For this review, take the finished solid that the model builds, in its own axes (mm). Give positions to 0.01 mm unless a question says otherwise; leave off trailing zeros. Write each loop counter-clockwise with the first axis right and the second up, starting at its lowest first coordinate (ties: lowest second). Pieces come first, ordered by that corner, then holes. Notation, with made-up numbers: (7.5, -33) -> (20.5, -33) arc R17 ccw to (20.5, -11) -> close; hole circle Ø10 at (88, 36). An arc over 180 degrees is marked (long way). Write item = value, one per line.
```python
from build123d import *

# Parameters (mm, degrees)
F0_R     = 1.5875
F1_DEPTH = 9
F3_W     = 12
F3_H     = 74
F4_DEPTH = 4


with BuildPart() as f1:
    # F0 (on Top) → F1 (new body)
    with BuildSketch(Plane.XY):
        Polygon((177, -37), (177, 37), (130, 37), (120, 47), (-120, 47), (-130, 37), (-177, 37), (-177, -37), (-130, -37), (-120, -47), (120, -47), (130, -37), align=None)
        with Locations((-135, -30)):
            Circle(F0_R, mode=Mode.SUBTRACT)
        with BuildLine():
            Line((-168, -8.5875), (-172, -8.5875))
            ThreePointArc((-172, -8.5875), (-173.5875, -7), (-172, -5.4125))
            Line((-172, -5.4125), (-168, -5.4125))
            ThreePointArc((-168, -5.4125), (-166.4125, -7), (-168, -8.5875))
        make_face(mode=Mode.SUBTRACT)
        with Locations((135, -30)):
            Circle(F0_R, mode=Mode.SUBTRACT)
        with BuildLine():
            Line((147, -21.4125), (151, -21.4125))
            ThreePointArc((151, -21.4125), (152.5875, -23), (151, -24.5875))
            Line((151, -24.5875), (147, -24.5875))
            ThreePointArc((147, -24.5875), (145.4125, -23), (147, -21.4125))
        make_face(mode=Mode.SUBTRACT)
        with BuildLine():
            Line((168, -13.4125), (172, -13.4125))
            ThreePointArc((172, -13.4125), (173.5875, -15), (172, -16.5875))
            Line((172, -16.5875), (168, -16.5875))
            ThreePointArc((168, -16.5875), (166.4125, -15), (168, -13.4125))
        make_face(mode=Mode.SUBTRACT)
        with BuildLine():
            Line((-168, 13.4125), (-172, 13.4125))
            ThreePointArc((-172, 13.4125), (-173.5875, 15), (-172, 16.5875))
            Line((-172, 16.5875), (-168, 16.5875))
            ThreePointArc((-168, 16.5875), (-166.4125, 15), (-168, 13.4125))
        make_face(mode=Mode.SUBTRACT)
        with BuildLine():
            Line((-147, 21.4125), (-151, 21.4125))
            ThreePointArc((-151, 21.4125), (-152.5875, 23), (-151, 24.5875))
            Line((-151, 24.5875), (-147, 24.5875))
            ThreePointArc((-147, 24.5875), (-145.4125, 23), (-147, 21.4125))
        make_face(mode=Mode.SUBTRACT)
        with Locations((-135, 30)):
            Circle(F0_R, mode=Mode.SUBTRACT)
        Polygon((120, 30), (130, 20), (130, -20), (120, -30), (-120, -30), (-130, -20), (-130, 20), (-120, 30), align=None, mode=Mode.SUBTRACT)
        with BuildLine():
            Line((168, 8.5875), (172, 8.5875))
            ThreePointArc((172, 8.5875), (173.5875, 7), (172, 5.4125))
            Line((172, 5.4125), (168, 5.4125))
            ThreePointArc((168, 5.4125), (166.4125, 7), (168, 8.5875))
        make_face(mode=Mode.SUBTRACT)
        with Locations((135, 30)):
            Circle(F0_R, mode=Mode.SUBTRACT)
    extrude(amount=F1_DEPTH)

    # F3 (on face) → F4 (cut)
    with BuildSketch(Plane.XY.offset(9)):
        with Locations((-171, 0)):
            Rectangle(F3_W, F3_H)
        with BuildLine():
            ThreePointArc((-168, -5.4125), (-166.4125, -7), (-168, -8.5875))
            Line((-168, -8.5875), (-172, -8.5875))
            ThreePointArc((-172, -8.5875), (-173.5875, -7), (-172, -5.4125))
            Line((-172, -5.4125), (-168, -5.4125))
        make_face(mode=Mode.SUBTRACT)
        with BuildLine():
            ThreePointArc((-168, 16.5875), (-166.4125, 15), (-168, 13.4125))
            Line((-168, 13.4125), (-172, 13.4125))
            ThreePointArc((-172, 13.4125), (-173.5875, 15), (-172, 16.5875))
            Line((-172, 16.5875), (-168, 16.5875))
        make_face(mode=Mode.SUBTRACT)
        with Locations((171, 0)):
            Rectangle(F3_W, F3_H)
        with BuildLine():
            ThreePointArc((168, -16.5875), (166.4125, -15), (168, -13.4125))
            Line((168, -13.4125), (172, -13.4125))
            ThreePointArc((172, -13.4125), (173.5875, -15), (172, -16.5875))
            Line((172, -16.5875), (168, -16.5875))
        make_face(mode=Mode.SUBTRACT)
        with BuildLine():
            ThreePointArc((168, 5.4125), (166.4125, 7), (168, 8.5875))
            Line((168, 8.5875), (172, 8.5875))
            ThreePointArc((172, 8.5875), (173.5875, 7), (172, 5.4125))
            Line((172, 5.4125), (168, 5.4125))
        make_face(mode=Mode.SUBTRACT)
    extrude(amount=-F4_DEPTH, mode=Mode.SUBTRACT)


solid = f1.part
```
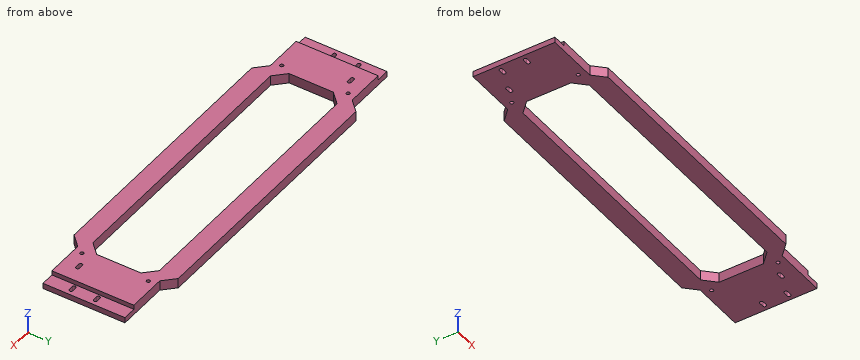
(1) Take a section at B-B (z = 6.75). Count the separate pieces of the cut face and the enclosed holes in it, plus the area to 3 significant figures.
Answers below:
separate_pieces = 1
enclosed_holes = 7
area = 13,900 mm^2
(2) To check wall thickness, follow probe 1 along Y at (x, z) = (-135, 3.75); probe 2 along X at (y, z) = (17, 1.5); probe 3 along Y at (x, z) = (-49.5, 3). State the ranges of each line that lie inside material, in increasing order.
Answers below:
probe_1 = -37 to -31.59, -28.41 to 28.41, 31.59 to 37
probe_2 = -177 to -130, 130 to 177
probe_3 = -47 to -30, 30 to 47
(3) Take a section at A-A (x = 93). Write out the cut boundary in (y, z), plus the area to 3 significant figures.
Answers below:
outline = (-47, 0) -> (-30, 0) -> (-30, 9) -> (-47, 9) -> close; (30, 0) -> (47, 0) -> (47, 9) -> (30, 9) -> close
area = 306 mm^2
(4) For pin 1 (5 mm diameter, centred on y = 11.5, z = 8, fed in from +X); pin 2 (1.2 mm diameter, centred on y = 15.5, z = 6.5, fed in from -X); pin 3 (8 mm diameter, centred on x = 31.5, y = -22.5, fed in from -Z); pin 4 (3.5 mm diameter, centred on x = -170.5, y = 9, fed in from +Z), all flat-tipped, find the tip position at first contact; note any pin that passes through.
Answers below:
pin_1 = 165
pin_2 = -165
pin_3 = through
pin_4 = 5
